Design review of the part built by this model. Coordinates are the model's own, in mm. A direction names the side the tool comes from. Coordinates: 2 decimals unless noted, no trailing zeros. Loops run counter-clockwise (first coordinate to the right, second up) from the corner with the lowest first, then second, coordinate; pieces in that order, holes last. Notation, with made-up numbers: (54, 17.25) - (102, 17.25) arc R32 ccw to (102, 55.25) - close; hole circle Ø9 at (5.5, -0.75). An arc over 180 degrees is marked (long way). Use one line per item in the form item = value. Start each with the question number.
(1) The part is to be moulded in two halves that separate along X. For faces 6 (the face through (21, 35, 0)), 7 (the face through (3, 39.5, -11)), 8 (the face through (-9, 40, 14)), say which applies: pulls with the +X half, pulls with the -X half, needs draft (parallel to the pull), parting line crosses it, or undercut.
(2) Clearance check with flat-ended pins moving along their axes: pin 1 Ø0.9 at (x, z) = (-15, -15) entering from +Y; pin 2 Ø6 at (x, y) = (0.5, 17) entering from +Z; pin 3 Ø3 at (x, z) = (10, 2.5) entering from +Y. State where each tip first meets the part, or that it passes through.
(3) For L1, parallel to Z at x = 0, y = 39.9; L2, parallel to Z at x = -15.5, y = 38.65; L3, parallel to Y at x = 16.5, z = 19.5, list the stretches that pass through material, from the lowest coordinate up.
(4) Tool access review of faces 1 (the face through (-17.9, 20.1, 17.9)), 2 (the face through (17.9, 20.1, 17.9)), 3 (the face through (0, 42, 5)), 4 (the face through (17.9, 20.1, -17.9)), 5 (the face through (-18.8, 30, -18.8)): name each direction out of +Z, -Z, +X, -X, +Y, -Y from which nothing blocks a thin tool from reaching the whole face with its end or side.
(5) Add section C-C (y = 53.5). State the section outline as (x, z) points.
Autodesk Inventor part; units mm, degrees
ref_plane "Work Plane1" through (0, 20, 0) normal (0, 1, 0) x (1, 0, 0)
ref_plane "YZ Plane" through (0, 0, 0) normal (1, 0, 0) x (0, 1, 0)
ref_plane "XZ Plane" through (0, 0, 0) normal (0, 1, 0) x (-1, 0, 0)
sketch "Sketch1" plane through (0, 0, 0) normal (0, 1, 0) x (-1, 0, 0)
  line L0 (-21, 21) -> (21, 21)
  line L1 (21, 21) -> (21, -21)
  line L2 (21, -21) -> (-21, -21)
  line L3 (-21, -21) -> (-21, 21)
  line L4 (-21, 21) -> (21, -21) construction
  line L5 (21, 21) -> (-21, -21) construction
  point P0 (0, 0)
  dimension "d0" = 42
  dimension "d1" = 42
extrude "Extrusion1" add sketch "Sketch1" along normal blind 40
ref_plane "Work Plane1" through (0, 20, 0) normal (0, 1, 0) x (1, 0, 0)
sketch "Sketch2" plane through (0, 40, 0) normal (0, 1, 0) x (1, 0, 0)
  line L0 (0, -38.0423) -> (-38.0423, 0)
  line L1 (-38.0423, 0) -> (0, 38.0423)
  line L2 (0, 38.0423) -> (38.0423, 0)
  line L3 (38.0423, 0) -> (0, -38.0423)
  line L4 (0, -38.0423) -> (0, 38.0423) construction
  line L5 (-38.0423, 0) -> (38.0423, 0) construction
  line L6 (-21, 21) -> (-21, -21)
  circle A0 centre (0, 0) radius 250
  dimension "d4" = 53.8
  dimension "d5" = 53.8
  dimension "d6" = 500
extrude "Extrusion2" cut sketch "Sketch2" against normal blind 10
sketch "Sketch3" plane through (0, 20, 0) normal (0, 1, 0) x (1, 0, 0)
  line L0 (-20.9, -20.9) -> (20.9, -20.9)
  line L1 (20.9, -20.9) -> (20.9, 20.9)
  line L2 (20.9, 20.9) -> (-20.9, 20.9)
  line L3 (-20.9, 20.9) -> (-20.9, -20.9)
  line L4 (-21, -21) -> (-21, -17.0423)
  line L5 (21, -21) -> (17.0423, -21)
  line L6 (21, 21) -> (21, 17.0423)
  line L7 (-21, 21) -> (-17.0423, 21)
  circle A0 centre (0, 0) radius 200
  dimension "d9" = 0.1
  dimension "d10" = 0.1
  dimension "d11" = 0.1
  dimension "d12" = 0.1
  dimension "d13" = 400
extrude "Extrusion3" cut sketch "Sketch3" along normal up to surface (10 mm away)
chamfer "Chamfer1" distance 6 angle 45 4 edges at (20.9, 25, 20.9) (20.9, 25, -20.9) (-20.9, 25, 20.9) (-20.9, 25, -20.9)
mirror "Mirror1" about plane through (0, 20, 0) normal (0, 1, 0) of "Extrusion3", "Extrusion2", "Chamfer1"
sketch "Sketch4" plane through (0, 40, 0) normal (0, 1, 0) x (1, 0, 0)
  circle A0 centre (0, 0) radius 11
  dimension "d19" = 22
extrude "Extrusion4" add sketch "Sketch4" along normal blind 2
sketch "Sketch5" plane through (0, 40, 0) normal (0, 1, 0) x (1, 0, 0)
  circle A0 centre (0, 0) radius 11
  line L0 (17.0423, -21) -> (21, -17.0423)
  line L1 (21, -17.0423) -> (21, 17.0423)
  line L2 (21, 17.0423) -> (17.0423, 21)
  line L3 (17.0423, 21) -> (-17.0423, 21)
  line L4 (-17.0423, 21) -> (-21, 17.0423)
  line L5 (-21, 17.0423) -> (-21, -17.0423)
  line L6 (-21, -17.0423) -> (-17.0423, -21)
  line L7 (-17.0423, -21) -> (17.0423, -21)
  circle A1 centre (0, 0) radius 16
  dimension "d22" = 32
extrude "Extrusion5" cut sketch "Sketch5" against normal blind 0.5 contours A1
sketch "Sketch6" plane through (0, 42, 0) normal (0, 1, 0) x (1, 0, 0)
  circle A0 centre (0, 0) radius 4.5
  dimension "d25" = 9
extrude "Extrusion6" cut sketch "Sketch6" against normal blind 2
sketch "Sketch7" plane through (0, 40, 0) normal (0, 1, 0) x (1, 0, 0)
  circle A0 centre (0, 0) radius 4
  dimension "d28" = 8
extrude "Extrusion7" add sketch "Sketch7" along normal blind 350
thread "Thread1"
chamfer "Chamfer2" distance 0.5 angle 45 1 edges at (-4, 390, 0)
sketch "Sketch8" plane through (0, 40, 0) normal (0, 1, 0) x (1, 0, 0)
  circle A0 centre (0, 0) radius 16 construction
  line L0 (17.0423, -21) -> (21, -17.0423) construction
  line L1 (21, -17.0423) -> (21, 17.0423) construction
  line L2 (21, 17.0423) -> (17.0423, 21) construction
  line L3 (17.0423, 21) -> (-17.0423, 21) construction
  line L4 (-17.0423, 21) -> (-21, 17.0423) construction
  line L5 (-21, 17.0423) -> (-21, -17.0423) construction
  line L6 (-21, -17.0423) -> (-17.0423, -21) construction
  line L7 (-17.0423, -21) -> (17.0423, -21) construction
  line L8 (-15.5, -15.5) -> (15.5, -15.5) construction
  line L9 (15.5, -15.5) -> (15.5, 15.5) construction
  line L10 (15.5, 15.5) -> (-15.5, 15.5) construction
  line L11 (-15.5, 15.5) -> (-15.5, -15.5) construction
  line L12 (-15.5, -15.5) -> (15.5, 15.5) construction
  line L13 (15.5, -15.5) -> (-15.5, 15.5) construction
  circle A1 centre (-15.5, 15.5) radius 1.5
  circle A2 centre (15.5, 15.5) radius 1.5
  circle A3 centre (15.5, -15.5) radius 1.5
  circle A4 centre (-15.5, -15.5) radius 1.5
  dimension "d36" = 31
  dimension "d37" = 31
  dimension "d38" = 3
  dimension "d39" = 3
  dimension "d40" = 3
  dimension "d41" = 3
extrude "Extrusion8" cut sketch "Sketch8" against normal blind 5
thread "Thread2"
pattern_circular "Circular Pattern1" count 4 over 360 about axis through (0, 40, 0) along (0, 1, 0) of "Extrusion8"
equation "\"d9\" = d10"
equation "\"d11\" = d10"
equation "\"d12\" = d10"
properties part number "linear_stepper_350mm"
Computed values:
q1.face_6 = pulls with the +X half
q1.face_7 = undercut
q1.face_8 = needs draft
q2.pin_1 = 35
q2.pin_2 = 20.9
q2.pin_3 = 42
q3.L1 = -21 to -16, -11 to 11, 16 to 21
q3.L2 = -21 to -17, -14 to 14, 17 to 21
q3.L3 = 0 to 10, 30 to 40
q4.face_1 = +Z, -X
q4.face_2 = +Z, +X
q4.face_3 = +Y
q4.face_4 = -Z, +X
q4.face_5 = none
q5.outline = circle Ø8 at (0, 0)
